```python
from build123d import *

# Parameters (mm, degrees)
SKIZZE2_W                       = 26
SKIZZE2_H                       = 26
AUFSATZ_LINEAR_AUSTRAGEN1_DEPTH = 16


with BuildPart() as part:
    # Skizze2 → Aufsatz-Linear austragen1 (new body)
    with BuildSketch(Plane(origin=(0, 0, 0), x_dir=(0, 1, 0), z_dir=(0, 0, 1))):
        Rectangle(SKIZZE2_W, SKIZZE2_H)
    extrude(amount=AUFSATZ_LINEAR_AUSTRAGEN1_DEPTH)

    # Skizze5 → Formsenkung für M3 Senkschraube mit Innensechskant1 (revolve, cut)
    with BuildSketch(Plane(origin=(0, 0, 16), x_dir=(0, -1, 0), z_dir=(1, 0, 0))):
        Polygon((0, 0), (0, 16), (1.7, 16), (1.7, 4.77), (3.47, 3), (3.47, 0), align=None)
    revolve(axis=Axis((0, 0, 22.35), (0, 0, -1)), mode=Mode.SUBTRACT)


solid = part.part
```
Could you check a few things on this model? Use its own coordinates, in mm. A direction names the side the tool comes from. Round coordinates to 2 decimals unless told otherwise and drop trailing zeros. Write each loop counter-clockwise with the first axis right and the second up, starting at its lowest first coordinate (ties: lowest second). Pieces come first, ordered by that corner, then holes. Notation, with made-up numbers: M 41.25,45.5 L 54.25,45.5 A21 ccw 54.25,56.5 Z; hole C -11,-2.5 d3. An arc over 180 degrees is marked long. Write each question's results on one line, items separated by ' | '. Start each with the question number.
1. On a 3-axis mill with a long thin cutter (end or side, diameter ignored), from which of +Z, -Z, +X, -X, +Y, -Y can I reach the whole of each face in a straight line? I mean faces 5 (the face through (-1.04, -3.31, 14.52)), 6 (the face through (0, -3, 0)). Say none if no direction works.
2. Thinking about a two-plate mould opening in Y: for faces 1 (the face through (13, 0, 8)), 2 (the face through (-1.795, 0.236, 11.341)), 3 (the face through (0, 13, 8)), 4 (the face through (0, -13, 8)), which applies, +Y half, -Y half, draft (parallel to the pull), parting line (faces both ways), or undercut?
3. I need wall thicknesses on L1, parallel to Y at x = 0, z = 15.3; L2, parallel to X at y = 0, z = 5. Which ranges of each line are inside material? Lowest first, please. Write a range as from..to.
4. I'm going to push a flat-ended pin straight in: pin 1 Ø3 at (x, y) = (0, 0) entering from -Z. Where does the tip first touch, or does it pass through?
5. Imagine slicing it at A-A on x = 0. List the corners of the cut face in (y, z) for me, and give its area (3 significant figures).
Result sheet:
1) face 5: +Z | face 6: -Z, +X, -X, +Y, -Y
2) face 1: draft | face 2: undercut | face 3: +Y half | face 4: -Y half
3) L1: y = -13..-3.47, 3.47..13 | L2: x = -13..-1.7, 1.7..13
4) pin 1: passes through
5) outline: M -13,0 L -1.7,0 L -1.7,11.23 L -3.47,13 L -3.47,16 L -13,16 Z; M 1.7,0 L 13,0 L 13,16 L 3.47,16 L 3.47,13 L 1.7,11.23 Z | area: 348 mm^2
